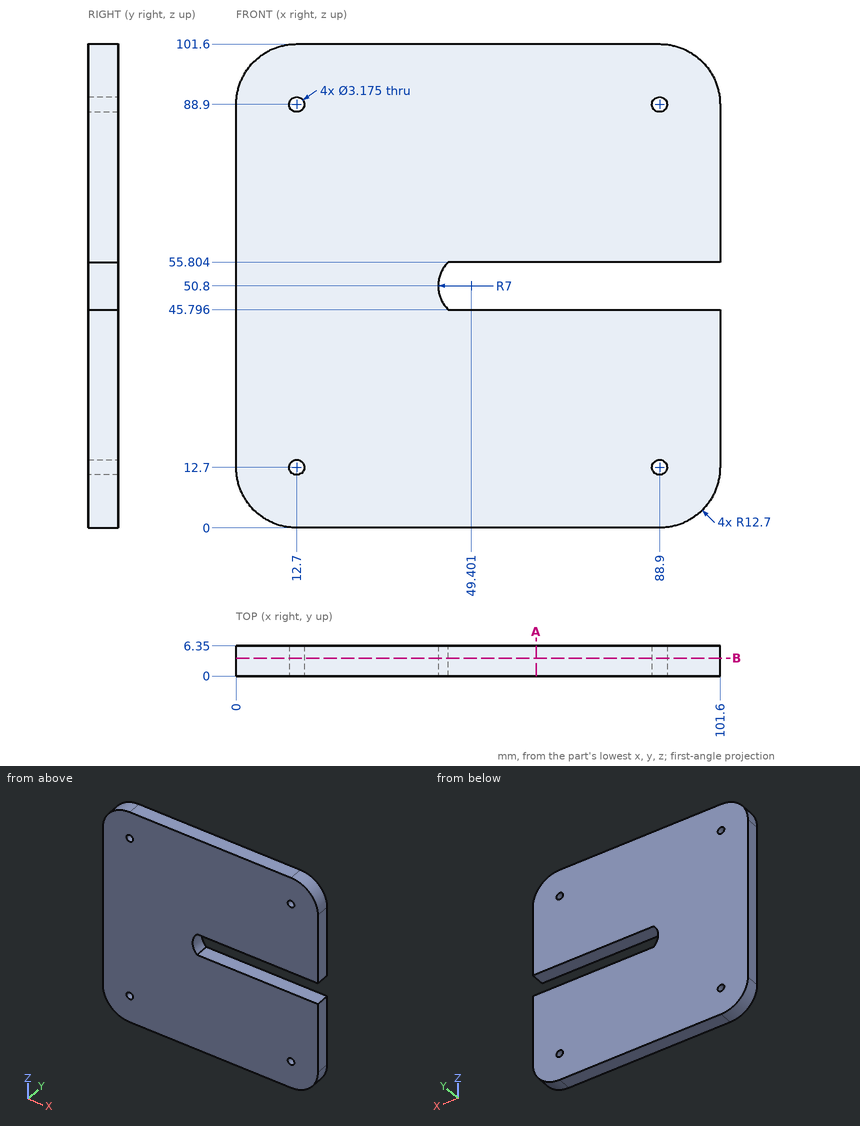
The drawing under review shows one solid part. Ordinate dimensions are in mm from its lowest x, y, z. Coordinates: 2 decimals unless noted, no trailing zeros. Write each loop counter-clockwise with the first axis right and the second up, starting at its lowest first coordinate (ties: lowest second). Pieces come first, ordered by that corner, then holes. Notation, with made-up numbers: M 75,-32.5 L 117,-32.5 A32 ccw 117,4.5 Z; hole C 44.5,-33.75 d9. An arc over 180 degrees is marked long. Put each result on its own line as item: value.
1) Add section A-A on x = 63. Give the boundary of the cut face in (y, z).
Computed:
outline: M 0,0 L 6.35,0 L 6.35,45.8 L 0,45.8 Z; M 0,55.8 L 6.35,55.8 L 6.35,101.6 L 0,101.6 Z
2) Add section B-B on y = 3.75. Give the boundary of the cut face in (x, z) (1 decimal), then the cut area to 3 significant figures.
Computed:
outline: M 0,12.7 A12.7 ccw 12.7,0 L 88.9,0 A12.7 ccw 101.6,12.7 L 101.6,45.8 L 44.5,45.8 A7 cw 44.5,55.8 L 101.6,55.8 L 101.6,88.9 A12.7 ccw 88.9,101.6 L 12.7,101.6 A12.7 ccw 0,88.9 Z; hole C 12.7,12.7 d3.2; hole C 12.7,88.9 d3.2; hole C 88.9,12.7 d3.2; hole C 88.9,88.9 d3.2
area: 9,570 mm2
3) Wall thickness on probe 1 along X at (y, z) = (2.25, 88.9); probe 2 along Z at (x, y) = (86.5, 5.5); probe 3 along Z at (x, y) = (96.5, 4) (1 decimal): over which ranges is each line inside the solid? List them lowest first. Write a range as [from, to].
Computed:
probe 1: x = [0, 11.11], [14.29, 87.31], [90.49, 101.6]
probe 2: z = [0, 45.8], [55.8, 101.6]
probe 3: z = [2.5, 45.8], [55.8, 99.1]
